Geometry: final body of the model. Coordinates: model frame, mm. A direction names the side the tool comes from. Coordinates: 2 decimals unless noted, no trailing zeros. Order: outer loops, then holes, each group sorted by start corner. A loop starts at its lowest first (then second) coordinate and runs counter-clockwise, first axis right, second up. Notation, with made-up numbers: M 65,15.25 L 90,15.25 A24 ccw 90,49.25 Z; hole C 73.5,63 d3. An arc over 180 degrees is marked long. Write item = value, one per line. Start each with the question number.
Autodesk Inventor part; units mm, degrees
ref_plane "YZ Plane" through (0, 0, 0) normal (1, 0, 0) x (0, 1, 0)
ref_plane "XZ Plane" through (0, 0, 0) normal (0, 1, 0) x (-1, 0, 0)
ref_plane "XY Plane" through (0, 0, 0) normal (0, 0, 1) x (1, 0, 0)
sketch "Sketch1" plane through (0, 0, 0) normal (0, 0, 1) x (1, 0, 0)
  circle A0 centre (36, 22) radius 1.25
  circle A1 centre (36, 22) radius 3
  arc A2 (0, 0) -> (36, 22) centre (4.7671, 32.6539) ccw construction
  arc A3 (-0.4334, -2.9685) -> (38.8394, 21.0315) centre (4.7671, 32.6539) ccw
  arc A4 (0.4334, 2.9685) -> (33.1606, 22.9685) centre (4.7671, 32.6539) ccw
  arc A5 (0.4334, 2.9685) -> (-0.4334, -2.9685) centre (0, 0) ccw
  arc A6 (38.8394, 21.0315) -> (33.1606, 22.9685) centre (36, 22) ccw
  point P0 (41.5332, 21.1583)
  point P1 (35.8668, 23.1312)
  point P2 (38.8394, 21.0315)
  point P3 (33.1606, 22.9685)
  dimension "d1" = 30
  dimension "d21" = 6
  dimension "d22" = 2.5
  dimension "d23" = 36
  dimension "d24" = 22
extrude "Extrusion1" add sketch "Sketch1" along normal blind 3
sketch "Sketch3" plane through (0, 0, 3) normal (0, 0, 1) x (1, 0, 0)
  arc A0 (-1, 0.1617) -> (1, -0.1304) centre (4.7671, 32.6539) ccw construction
  arc A1 (-1.8738, -4.7614) -> (0.4292, -5.0977) centre (4.7671, 32.6539) ccw
  arc A2 (-0.1262, 5.0848) -> (1.5708, 4.8369) centre (4.7671, 32.6539) ccw
  arc A3 (-0.1262, 5.0848) -> (-1.8738, -4.7614) centre (-1, 0.1617) ccw
  arc A4 (0.4292, -5.0977) -> (1.5708, 4.8369) centre (1, -0.1304) ccw
  arc A5 (-0.4334, -2.9685) -> (38.8394, 21.0315) centre (4.7671, 32.6539) ccw
  point P0 (0, 0)
  dimension "d31" = 10
  dimension "d32" = 1
  dimension "d33" = 1
extrude "Extrusion3" add sketch "Sketch3" against normal blind 3
sketch "Sketch4" plane through (0, 0, 3) normal (0, 0, -1) x (1, 0, 0)
  arc A0 (-1.8738, 4.7614) -> (-0.1262, -5.0848) centre (-1, -0.1617) ccw
  arc A1 (0.4292, 5.0977) -> (-1.8738, 4.7614) centre (4.7671, -32.6539) ccw
  arc A2 (1.5708, -4.8369) -> (-0.1262, -5.0848) centre (4.7671, -32.6539) ccw
  arc A3 (1, 0.1304) -> (-1, -0.1617) centre (4.7671, -32.6539) ccw construction
  arc A4 (0.7146, 2.6141) -> (-1.4369, 2.2998) centre (4.7671, -32.6539) ccw
  arc A5 (1.2854, -2.3532) -> (-0.5631, -2.6232) centre (4.7671, -32.6539) ccw
  arc A6 (1.2854, -2.3532) -> (0.7146, 2.6141) centre (1, 0.1304) ccw
  arc A7 (-1.4369, 2.2998) -> (-0.5631, -2.6232) centre (-1, -0.1617) ccw
  arc A8 (33.1606, -22.9685) -> (5.1514, -2.6563) centre (4.7671, -32.6539) ccw
  arc A9 (33.1606, -22.9685) -> (38.8394, -21.0315) centre (36, -22) ccw
  arc A10 (38.8394, -21.0315) -> (4.8288, 3.3461) centre (4.7671, -32.6539) ccw
  arc A11 (4.8288, 3.3461) -> (0.4292, 5.0977) centre (1, 0.1304) ccw
  arc A12 (1.5708, -4.8369) -> (5.1514, -2.6563) centre (1, 0.1304) ccw
  arc A13 (1.3767, -3.148) -> (-0.4233, -3.4109) centre (4.7671, -32.6539) ccw
  arc A14 (1.3767, -3.148) -> (0.6233, 3.4088) centre (1, 0.1304) ccw
  arc A15 (0.6233, 3.4088) -> (-1.5767, 3.0875) centre (4.7671, -32.6539) ccw
  arc A16 (-1.5767, 3.0875) -> (-0.4233, -3.4109) centre (-1, -0.1617) ccw
  point P0 (0, 0)
  dimension "d43" = 5
  dimension "d52" = 0.8
extrude "Extrusion4" cut sketch "Sketch4" along normal through all contours A6 A5 A7 A4
sketch "Sketch5" plane through (0, 0, 3) normal (0, 0, 1) x (1, 0, 0)
  circle A0 centre (36, 22) radius 1.25
  arc A1 (0, 0) -> (36, 22) centre (4.7671, 32.6539) ccw construction
  arc A2 (39.7686, 20.6592) -> (32.2314, 23.3408) centre (36, 22) ccw
  arc A3 (31.9418, 22.5269) -> (39.479, 19.8452) centre (35.7104, 21.1861) ccw
  line L0 (35.0504, 21.4307) -> (36.2779, 20.9758)
  line L1 (37.5646, 21.4663) -> (34.5144, 22.5068)
  line L2 (31.9418, 22.5269) -> (32.2314, 23.3408)
  line L3 (39.479, 19.8452) -> (39.7686, 20.6592)
  circle A4 centre (36, 22) radius 1.8
  dimension "d44" = 8
  dimension "d46" = 1.5
  dimension "d47" = 3.6
extrude "Extrusion5" cut sketch "Sketch5" against normal up to surface (3 mm away) contours A4
extrude "Extrusion6" add sketch "Sketch5" against normal up to surface (3 mm away) contours L3 A3 L2 A2
extrude "Extrusion7" cut sketch "Sketch4" along normal blind 1 contours A13 A16 A15 A14
sketch "Sketch6" plane through (0, 0, 0) normal (0, 0, -1) x (-1, 0, 0)
  circle A0 centre (-36, 22) radius 1.8
  arc A1 (-37.4644, 17.5911) -> (-4.8288, -3.3461) centre (-4.7671, 32.6539) ccw
  arc A2 (-4.8288, -3.3461) -> (-0.4292, -5.0977) centre (-1, -0.1304) ccw
  arc A3 (-0.4292, -5.0977) -> (1.8738, -4.7614) centre (-4.7671, 32.6539) ccw
  arc A4 (1.8738, -4.7614) -> (0.1262, 5.0848) centre (1, 0.1617) ccw
  arc A5 (-1.5708, 4.8369) -> (0.1262, 5.0848) centre (-4.7671, 32.6539) ccw
  arc A6 (-1.5708, 4.8369) -> (-5.1514, 2.6563) centre (-1, -0.1304) ccw
  arc A7 (-31.9221, 19.9021) -> (-5.1514, 2.6563) centre (-4.7671, 32.6539) ccw
  arc A8 (-31.9221, 19.9021) -> (-31.9418, 22.5269) centre (-35.7104, 21.1861) ccw
  line L0 (-31.9418, 22.5269) -> (-32.2314, 23.3408)
  arc A9 (-32.2314, 23.3408) -> (-39.7686, 20.6592) centre (-36, 22) ccw
  line L1 (-39.7686, 20.6592) -> (-39.479, 19.8452)
  arc A10 (-39.479, 19.8452) -> (-37.4644, 17.5911) centre (-35.7104, 21.1861) ccw
  arc A11 (-0.7146, -2.6141) -> (1.4369, -2.2998) centre (-4.7671, 32.6539) ccw
  arc A12 (-1.2854, 2.3532) -> (-0.7146, -2.6141) centre (-1, -0.1304) ccw
  arc A13 (-1.2854, 2.3532) -> (0.5631, 2.6232) centre (-4.7671, 32.6539) ccw
  arc A14 (1.4369, -2.2998) -> (0.5631, 2.6232) centre (1, 0.1617) ccw
  arc A15 (-32.2314, 23.3408) -> (-39.7686, 20.6592) centre (-36, 22) ccw
  arc A16 (-32.2466, 20.6173) -> (-32.2314, 23.3408) centre (-36, 22) ccw
  arc A17 (-31.9221, 19.9021) -> (-5.1514, 2.6563) centre (-4.7671, 32.6539) ccw
  arc A18 (-32.2466, 20.6173) -> (-31.9221, 19.9021) centre (-4.7671, 32.6539) ccw
  arc A19 (-31.9221, 19.9021) -> (-5.1514, 2.6563) centre (-4.7671, 32.6539) ccw
  point P0 (0, 0)
extrude "Extrusion8" cut sketch "Sketch6" against normal up to surface (3 mm away) contours L0 A8 A18 A16
Item 1: Section query A-A on y = 22. Output: boundary loops of the cut face in (x, z), and give its area (3 significant figures).
Item 2: Reachability of faces 1 (the cylindrical face through (3.63, 4.12, 1.52)), 2 (the cylindrical face through (3.477, -0.47, 1.014)), 3 (the flat face through (0, -3, 2)), 4 (the cylindrical face through (32, 22, 1)) from +Z, -Z, +X, -X, +Y, -Y: full face, straight path, thin tool, end or side. Return the list, or none.
Item 3: Section query B-B on x = 36. Output: boundary loops of the cut face in (y, z), and give its area (3 significant figures).
Item 4: Section query D-D on y = 0. Output: boundary loops of the cut face in (x, z), and give its area (3 significant figures).
Item 5: Draft query along Y for faces 5 (the cylindrical face through (-0.741, -4.945, 1.521)), 6 (the cylindrical face through (-5.903, 1.144, 1.521)), 7 (the cylindrical face through (36.968, 23.518, 1.521)). Return one class per face: pulls with the +Y half, pulls with the -Y half, needs draft (parallel to the pull), parting line crosses it, or undercut.
Item 6: Section query C-C on z = 1.15. Output: boundary loops of the cut face in (x, y), and give its area (3 significant figures).
Item 7: First-contact query: pin 1 (12 mm diameter, centred on x = 20.5, y = 21.5, fed in from -Z); pin 2 (1.5 mm diameter, centred on x = 21, z = 0.5, fed in from -Y); pin 3 (1 mm diameter, centred on x = 17.5, z = 2.5, fed in from -Y). Flat tips, straight axial feed; report the tip coordinate or a pass-through.
Item 8: Material intervals for probe 1 along Y at (x, z) = (36, 1.1); probe 2 along Y at (x, z) = (1.5, 0.95); probe 3 along X at (y, z) = (1, 0.1), sorted ascending. Write a range as [from, to].
Ans:
q1.outline = M 32,0 L 34.2,0 L 34.2,3 L 32,3 Z; M 37.8,0 L 40,0 L 40,3 L 37.8,3 Z
q1.area = 13.2 mm^2
q2.face_1 = +Z, -Z, +Y
q2.face_2 = +Z, -Z
q2.face_3 = +Z
q2.face_4 = +Z, -Z, -X
q3.outline = M 14.75,0 L 20.2,0 L 20.2,3 L 14.75,3 Z; M 23.8,0 L 26,0 L 26,3 L 23.8,3 Z
q3.area = 22.9 mm^2
q4.outline = M -6,0 L -3.49,0 L -3.49,2 L -4.3,2 L -4.3,3 L -6,3 Z; M 3.5,0 L 19.92,0 L 19.92,3 L 4.3,3 L 4.3,2 L 3.5,2 Z
q4.area = 55.2 mm^2
q5.face_5 = pulls with the -Y half
q5.face_6 = parting line crosses it
q5.face_7 = undercut
q6.outline = M -1.87,-4.76 A37.92 ccw 0.43,-5.1 A5 ccw 4.83,-3.35 A36 ccw 37.46,17.59 A4 ccw 39.48,19.85 L 39.77,20.66 A4 ccw 32.23,23.34 A4 ccw 32.25,20.62 A29.98 cw 31.92,19.9 A30 cw 5.15,2.66 A5 ccw 1.57,4.84 A28.04 cw -0.13,5.08 A5 ccw Z; hole M -1.44,-2.3 A35.44 ccw 0.71,-2.61 A2.5 ccw 1.29,2.35 A30.49 cw -0.56,2.62 A2.5 ccw Z; hole C 36,22 d3.6
q6.area = 329 mm^2
q7.pin_1 = through
q7.pin_2 = 0.15
q7.pin_3 = -1.2
q8.probe_1 = [14.75, 20.2], [23.8, 26]
q8.probe_2 = [-5.11, -2.58], [2.32, 4.85]
q8.probe_3 = [-5.93, -3.36], [3.23, 21.91]
